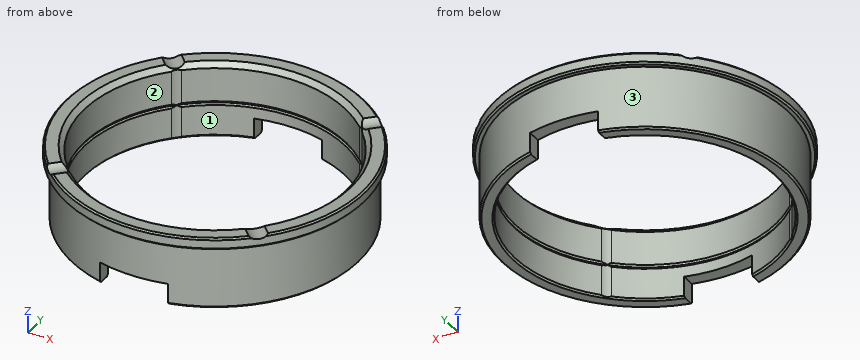
```python
from build123d import *

# Parameters (mm, degrees)
SKETCH33_MESH_154_R                  = 4.25
CUT_EXTRUDE1_DEPTH                   = 69.616925755
SKETCH34_MESH_158_R                  = 3.9
EXTRUDE21_CUT_159_DEPTH              = 22.5
CIRPATTERN1_COUNT                    = 4
CUT_EXTRUDE11_REACH                  = 69.103
CUT_EXTRUDE11_END_RADIUS             = 44
SKETCH35_MESH_161_W                  = 20.9
SKETCH35_MESH_161_H                  = 6.5
CUT_EXTRUDE11_DIRECTION_2_REACH      = 69.103
CUT_EXTRUDE11_DIRECTION_2_END_RADIUS = 44


with BuildPart() as part:
    # Sketch32 (Mesh)_152 → Revolve1 (revolve)
    with BuildSketch(Plane(origin=(0, 0, 0), x_dir=(0, 0, -1), z_dir=(1, 0, 0)), mode=Mode.PRIVATE) as revolve1_sk:
        Polygon((-16.55, -40.05), (-6.106217783, -40.05), (-5.5, -40.4), (-4.893782217, -40.05), (4.5, -40.05), (5, -40.55), (5, -43.5), (4.5, -44), (-14.45, -44), (-14.45, -45.2), (-14.95, -45.7), (-17.55, -45.7), (-18.05, -45.2), (-18.05, -41.55), align=None)
    revolve(revolve1_sk.sketch.rotate(Axis((0, 0, 0), (0, 0, 1)), 180), axis=Axis((0, 0, 0), (0, 0, 1)))

    # Sketch33 (Mesh)_154 → Cut-Extrude1 (cut, through all)
    with BuildSketch(Plane.XY.offset(18.05)):
        with Locations((-25.455844123, 25.455844123)):
            Circle(SKETCH33_MESH_154_R)
    cut_extrude1 = extrude(amount=-CUT_EXTRUDE1_DEPTH, mode=Mode.SUBTRACT)

    # Sketch34 (Mesh)_158 → Extrude21 (Cut)_159 (cut, symmetric)
    with BuildSketch(Plane(origin=(-28.319626587, 28.319626587, 0), x_dir=(-0.7071067811865464, -0.7071067811865488, 0), z_dir=(0.7071067811865488, -0.7071067811865464, 0))):
        with Locations((0, -20.9)):
            Circle(SKETCH34_MESH_158_R)
    extrude21_cut_159 = extrude(amount=EXTRUDE21_CUT_159_DEPTH, both=True, mode=Mode.SUBTRACT)

    # CirPattern1: Cut-Extrude1, Extrude21 (Cut)_159 ×4 about axis
    cirpattern1_axis = Axis((0, 0, 0), (0, 0, 1))
    add([cut_extrude1.rotate(cirpattern1_axis, i * 360 / CIRPATTERN1_COUNT) for i in range(1, CIRPATTERN1_COUNT)], mode=Mode.SUBTRACT)
    add([extrude21_cut_159.rotate(cirpattern1_axis, i * 360 / CIRPATTERN1_COUNT) for i in range(1, CIRPATTERN1_COUNT)], mode=Mode.SUBTRACT)

    # Cut-Extrude11: up to this cylinder (the profile starts inside it)
    cut_extrude11_end = Plane(origin=(0, 0, -1.75), z_dir=(0, 0, -1)) * Cylinder(CUT_EXTRUDE11_END_RADIUS, 227.206, mode=Mode.PRIVATE)
    # Sketch35 (Mesh)_161 → Cut-Extrude11 (cut, up to the surface)
    with BuildSketch(Plane(origin=(0, 0, 0), x_dir=(1, 0, 0), z_dir=(0, 1, 0)), mode=Mode.PRIVATE) as cut_extrude11_sk1:
        with Locations((0, 1.75)):
            Rectangle(SKETCH35_MESH_161_W, SKETCH35_MESH_161_H)
    cut_extrude11_tool1 = extrude(cut_extrude11_sk1.sketch, amount=CUT_EXTRUDE11_REACH, mode=Mode.PRIVATE) & cut_extrude11_end
    add(cut_extrude11_tool1.solids().sort_by_distance((0, 0, -1.75))[0], mode=Mode.SUBTRACT)

    # Cut-Extrude11 direction 2: up to this cylinder (the profile starts inside it)
    cut_extrude11_direction_2_end = Plane(origin=(0, 0, -1.75), z_dir=(0, 0, -1)) * Cylinder(CUT_EXTRUDE11_DIRECTION_2_END_RADIUS, 227.206, mode=Mode.PRIVATE)
    # Sketch35 (Mesh)_161 → Cut-Extrude11 direction 2 (cut, up to the surface)
    with BuildSketch(Plane(origin=(0, 0, 0), x_dir=(1, 0, 0), z_dir=(0, 1, 0)), mode=Mode.PRIVATE) as cut_extrude11_direction_2_sk1:
        with Locations((0, 1.75)):
            Rectangle(SKETCH35_MESH_161_W, SKETCH35_MESH_161_H)
    cut_extrude11_direction_2_tool1 = extrude(cut_extrude11_direction_2_sk1.sketch, amount=-CUT_EXTRUDE11_DIRECTION_2_REACH, mode=Mode.PRIVATE) & cut_extrude11_direction_2_end
    add(cut_extrude11_direction_2_tool1.solids().sort_by_distance((0, 0, -1.75))[0], mode=Mode.SUBTRACT)


solid = part.part
```
Geometry: final body of the model. Coordinates: model frame, mm. Face numbers are marked on the shaded views. Coordinates: 2 decimals unless noted, no trailing zeros. Loops run counter-clockwise (first coordinate to the right, second up) from the corner with the lowest first, then second, coordinate; pieces in that order, holes last. Notation, with made-up numbers: (-21.5, -17.5) -> (-17.5, -17.5) arc R20 ccw to (-17.5, -4.5) -> close; hole circle Ø5 at (64.25, 61.25). An arc over 180 degrees is marked (long way). Use a Markdown table: item, result. Add a question column.
(1) Section query A-A, the plane z = -0.75. Return loops of the section in (x, y), plus the area to 3 significant figures.
(2) Section query B-B, the plane y = 0. Return loops of the section in (x, z), plus the area to 3 significant figures.
(3) Section query C-C, the plane x = 0. Return loops of the section in (y, z), plus the area to 3 significant figures.
(4) Line query: line 1 along Y through (x, z) = (17, 0.5); line 2 along Y through (x, z) = (-23.5, 1); line 3 along Z through (x, y) = (-19.5, 39.5). Output: solid intervals per line, ascending.
(5) Mould query, pull axis Y, two halves, no side actions, for the marked faces 1, 2 and 3. Classes: pulls with the +Y half, pulls with the -Y half, needs draft (parallel to the pull), parting line crosses it, or undercut.
(6) Pin query (flat end, axial travel): pin 1 Ø6 at (x, z) = (-23.5, 14.5) entering from +Y; pin 2 Ø4.5 at (y, z) = (-41.5, -2) entering from +X; pin 3 Ø4.5 at (x, y) = (-1, 40.5) entering from -Z. Return the tip coordinate at first contact, or that it passes through.
Answer:
| question | item | result |
|---|---|---|
| 1 | outline | (-29.26, -27.34) arc R40.05 cw to (-29.26, 27.34) arc R4.25 cw to (-27.34, 29.26) arc R40.05 cw to (-10.45, 38.66) -> (-10.45, 42.74) arc R44 ccw to (-10.45, -42.74) -> (-10.45, -38.66) arc R40.05 cw to (-27.34, -29.26) arc R4.25 cw to start; (10.45, -42.74) arc R44 ccw to (10.45, 42.74) -> (10.45, 38.66) arc R40.05 cw to (27.34, 29.26) arc R4.25 cw to (29.26, 27.34) arc R40.05 cw to (29.26, -27.34) arc R4.25 cw to (27.34, -29.26) arc R40.05 cw to (10.45, -38.66) -> close |
| 1 | area | 875 mm^2 |
| 2 | outline | (-45.7, 14.95) -> (-45.2, 14.45) -> (-44, 14.45) -> (-44, -4.5) -> (-43.5, -5) -> (-40.55, -5) -> (-40.05, -4.5) -> (-40.05, 4.89) -> (-40.4, 5.5) -> (-40.05, 6.11) -> (-40.05, 16.55) -> (-41.55, 18.05) -> (-45.2, 18.05) -> (-45.7, 17.55) -> close; (40.05, -4.5) -> (40.55, -5) -> (43.5, -5) -> (44, -4.5) -> (44, 14.45) -> (45.2, 14.45) -> (45.7, 14.95) -> (45.7, 17.55) -> (45.2, 18.05) -> (41.55, 18.05) -> (40.05, 16.55) -> (40.05, 6.11) -> (40.4, 5.5) -> (40.05, 4.89) -> close |
| 2 | area | 191 mm^2 |
| 3 | outline | (-45.7, 14.95) -> (-45.2, 14.45) -> (-44, 14.45) -> (-44, 1.5) -> (-40.05, 1.5) -> (-40.05, 4.89) -> (-40.4, 5.5) -> (-40.05, 6.11) -> (-40.05, 16.55) -> (-41.55, 18.05) -> (-45.2, 18.05) -> (-45.7, 17.55) -> close; (40.05, 1.5) -> (44, 1.5) -> (44, 14.45) -> (45.2, 14.45) -> (45.7, 14.95) -> (45.7, 17.55) -> (45.2, 18.05) -> (41.55, 18.05) -> (40.05, 16.55) -> (40.05, 6.11) -> (40.4, 5.5) -> (40.05, 4.89) -> close |
| 3 | area | 140 mm^2 |
| 4 | line 1 | y = -40.58 to -36.26, 36.26 to 40.58 |
| 4 | line 2 | y = -37.2 to -32.43, 32.43 to 37.2 |
| 4 | line 3 | z = 14.45 to 18.05 |
| 5 | face 1 | undercut |
| 5 | face 2 | undercut |
| 5 | face 3 | parting line crosses it |
| 6 | pin 1 | stops at y = 40.83 |
| 6 | pin 2 | stops at x = 19.89 |
| 6 | pin 3 | stops at z = 1.5 |
